Input: dimensioned drawing with shaded views. Units: mm. Origin: part minimum x, y, z. A direction names the side the tool comes from. Give positions to 0.01 mm unless a question says otherwise; leave off trailing zeros. Loops run counter-clockwise (first coordinate to the right, second up) from the corner with the lowest first, then second, coordinate; pieces in that order, holes last.
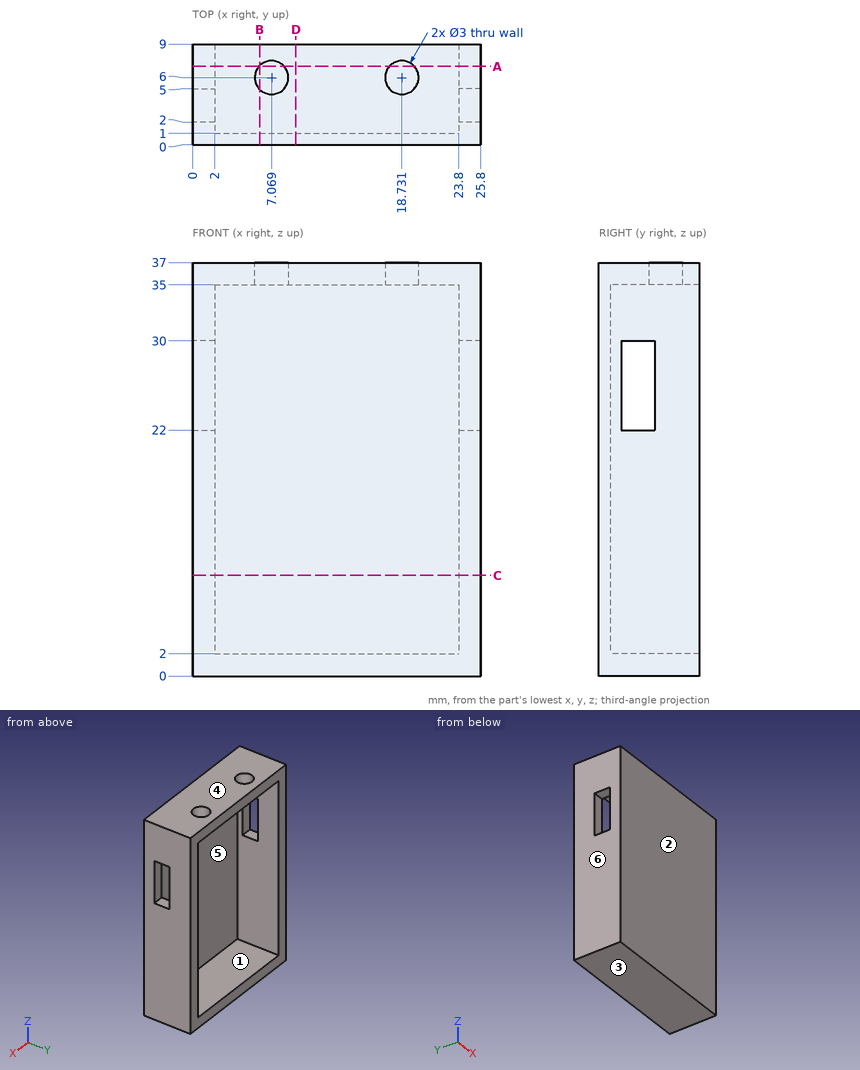
(1) Ray query, line 1 along Z through (x, y) = (16, 8.25); line 2 along Z through (x, y) = (1.5, 3.75); line 3 along Y through (x, z) = (11, 14). Return the intervals inside material, ascending.
A:
line 1: z = 0 to 2, 35 to 37
line 2: z = 0 to 22, 30 to 37
line 3: y = 0 to 1
(2) First-contact query: pin 1 (1.8 mm diameter, centred on x = 18.73, y = 6, fed in from +Z); pin 2 (2 mm diameter, centred on x = 17.5, z = 6.5, fed in from +Y); pin 3 (1 mm diameter, centred on y = 3, z = 28.5, fed in from -X). Flat tips, straight axial feed; report the tip coordinate or a pass-through.
A:
pin 1: stops at z = 2
pin 2: stops at y = 1
pin 3: passes through
(3) Section A-A, the plane y = 7. Return the cut outline in (x, z).
A:
outline: (0, 0) - (25.8, 0) - (25.8, 37) - (19.85, 37) - (19.85, 35) - (23.8, 35) - (23.8, 2) - (2, 2) - (2, 35) - (5.95, 35) - (5.95, 37) - (0, 37) - close; (8.19, 35) - (17.61, 35) - (17.61, 37) - (8.19, 37) - close
(4) Section D-D, the plane x = 9.25. Return the cut outline in (y, z), then the cut area to 3 significant figures.
A:
outline: (0, 0) - (9, 0) - (9, 2) - (1, 2) - (1, 35) - (9, 35) - (9, 37) - (0, 37) - close
area: 69.0 mm2
(5) Section C-C, the plane z = 9. Return the cut outline in (x, y), then the cut area to 3 significant figures.
A:
outline: (0, 0) - (25.8, 0) - (25.8, 9) - (23.8, 9) - (23.8, 1) - (2, 1) - (2, 9) - (0, 9) - close
area: 57.8 mm2
(6) Reachability of the marked faces 1 and 2 from +Z, -Z, +X, -X, +Y, -Y: full face, straight path, thin tool, end or side. Return the list, or none.
A:
face 1: +Y
face 2: +Z, -Z, +X, -X, -Y
(7) Section B-B, the plane x = 6. Return the cut outline in (y, z).
A:
outline: (0, 0) - (9, 0) - (9, 2) - (1, 2) - (1, 35) - (4.95, 35) - (4.95, 37) - (0, 37) - close; (7.05, 35) - (9, 35) - (9, 37) - (7.05, 37) - close
(8) Mould query, pull axis Z, two halves, no side actions, for the marked faces 3, 4, 5 and 6. Classes: pulls with the +Z half, pulls with the -Z half, needs draft (parallel to the pull), parting line crosses it, or undercut.
A:
face 3: pulls with the -Z half
face 4: pulls with the +Z half
face 5: undercut
face 6: needs draft
